Model file for the job. Use its own axes, mm. A direction names the side the tool comes from. Round coordinates to 2 decimals unless told otherwise and drop trailing zeros. Order: outer loops, then holes, each group sorted by start corner. A loop starts at its lowest first (then second) coordinate and runs counter-clockwise, first axis right, second up. Notation, with made-up numbers: (22, -23.75) -> (41, -23.75) arc R18 cw to (41, -7.75) -> close; hole circle Ø1 at (64.5, 57). An arc over 180 degrees is marked (long way). Put each result on its own line as item: value. Start each with the question number.
Q1. Pull direction Y, two halves, no side cores. Call faces 5 (the face through (-0.986, -4.714, -213.506)), 6 (the face through (44.15, 50.3, 3.4)), 7 (the face through (44.067, 47.942, 3.395)), 8 (the face through (-0.986, -4.714, 226.494)): released by +Y, released by -Y, zero draft, split by the parting line, or undercut.
Q2. Flat gauge pins, fed straight in: P1, Ø11, axis at x = 141.5, y = 69, coming from the +Z side; P2, Ø1.6, axis at y = 73.5, z = -232.5, coming from the +X side; P3, Ø15, axis at y = -5, z = 220, coming from the +X side. Where does each tip first touch, or does it go through?
Q3. Probe L1, parallel to Z at x = -0.85, y = -7.5; L2, parallel to X at y = 16.5, z = 79; L3, parallel to Y at x = -0.9, z = -220. List the from-to ranges inside material, lowest first.
Q4. Cut at B-B, the plane x = 121.5. List the corners of the cut face in (y, z).
Q5. Cut at A-A, the plane z = 148. List the corners of the cut face in (x, y).
Q6. Cut at C-C, the plane y = 38. List the corners of the cut face in (x, z).
Q7. 3-axis set-ups, long thin cutter, end or side, ignore diameter. For faces 1 (the face through (142.5, 67.9, -222.5)), 2 (the face through (0, -4, 3)), 3 (the face through (110, 72.152, 3)), 4 (the face through (142.5, 67.9, 222.5)): which of +Z, -Z, +X, -X, +Y, -Y reach the whole face in a straight line?
from build123d import *

# Parameters (mm, degrees)
BASIS_BLECH1_DEPTH               = 242.5
SKIZZE4_W                        = 22
SKIZZE4_H                        = 20
SCHNITT_LINEAR_AUSTRAGEN1_DEPTH  = 303.852114579
F_7_0_7_DURCHMESSER_BOHRUNG1_D   = 7
F_13_0_13_DURCHMESSER_BOHRUNG1_D = 13
F_7_0_7_DURCHMESSER_BOHRUNG2_D   = 7


# Sheet-metal steps are written as plain solids
with BuildPart() as part:
    # Skizze1 → Basis-Blech1 (new, symmetric)
    with BuildSketch(Plane.XY):
        with BuildLine():
            Line((0, -22.5), (0, 15.57179677))
            ThreePointArc((0, 15.57179677), (1.607695155, 21.57179677), (6, 25.964101615))
            Line((6, 25.964101615), (83.215390309, 70.544427996))
            ThreePointArc((83.215390309, 70.544427996), (86.109561768, 71.743233066), (89.215390309, 72.15212315))
            Line((89.215390309, 72.15212315), (132.216414533, 72.15212315))
            ThreePointArc((132.216414533, 72.15212315), (135.824884128, 71.596726559), (139.09933177, 69.981947682))
            Line((139.09933177, 69.981947682), (152.383040886, 60.680594423))
            Line((152.383040886, 60.680594423), (153.530193758, 62.318898512))
            Line((153.530193758, 62.318898512), (140.246484642, 71.62025177))
            ThreePointArc((140.246484642, 71.62025177), (136.426295727, 73.504160461), (132.216414533, 74.15212315))
            Line((132.216414533, 74.15212315), (89.215390309, 74.15212315))
            ThreePointArc((89.215390309, 74.15212315), (85.591923678, 73.675084718), (82.215390309, 72.276478803))
            Line((82.215390309, 72.276478803), (5, 27.696152423))
            ThreePointArc((5, 27.696152423), (-0.124355653, 22.57179677), (-2, 15.57179677))
            Line((-2, 15.57179677), (-2, -22.5))
            Line((-2, -22.5), (0, -22.5))
        make_face()
    extrude(amount=BASIS_BLECH1_DEPTH, both=True)

    # Skizze4 → Schnitt-Linear austragen1 (cut, through all)
    with BuildSketch(Plane(origin=(0, 74.15212315, 0), x_dir=(1, 0, 0), z_dir=(0, 1, 0))):
        with Locations((142.530193758, 232.5)):
            Rectangle(SKIZZE4_W, SKIZZE4_H)
        with Locations((142.530193758, -232.5)):
            Rectangle(SKIZZE4_W, SKIZZE4_H)
    extrude(amount=-SCHNITT_LINEAR_AUSTRAGEN1_DEPTH, mode=Mode.SUBTRACT)

    # Ø7.0 (7) Durchmesser Bohrung1 (through all)
    with Locations(Plane(origin=(-2, 72.15212315, 0), x_dir=(0, -1, 0), z_dir=(-1, 0, 0))):
        with Locations((79.65212315, 235), (79.65212315, -235)):
            Hole(F_7_0_7_DURCHMESSER_BOHRUNG1_D / 2)

    # Ø13.0 (13) Durchmesser Bohrung1 (through all)
    with Locations(Plane.ZY.offset(2)):
        with Locations((-220, -5), (220, -5)):
            Hole(F_13_0_13_DURCHMESSER_BOHRUNG1_D / 2)

    # Ø7.0 (7) Durchmesser Bohrung2 (through all)
    with Locations(Plane(origin=(79.790191976, 113.952203628, 0), x_dir=(0, 0, -1), z_dir=(0.5735764363510463, 0.8191520442889918, 0))):
        with Locations((0, -83.019920352), (-100, -83.019920352), (-200, -83.019920352), (100, -83.019920352), (200, -83.019920352)):
            Hole(F_7_0_7_DURCHMESSER_BOHRUNG2_D / 2)


solid = part.part
Ans:
1. face 5: undercut
1. face 6: released by +Y
1. face 7: released by -Y
1. face 8: undercut
2. P1: stops at z = 222.5
2. P2: stops at x = 131.53
2. P3: stops at x = 0
3. L1: z = -242.5 to -238.5, -231.5 to -226, -214 to 214, 226 to 231.5, 238.5 to 242.5
3. L2: x = -1.97 to 0.04
3. L3: y = -22.5 to -11.5, 1.5 to 21.01
4. outline: (72.15, -242.5) -> (74.15, -242.5) -> (74.15, 242.5) -> (72.15, 242.5) -> close
5. outline: (-2, -22.5) -> (0, -22.5) -> (0, 15.57) arc R12 cw to (6, 25.96) -> (83.22, 70.54) arc R12 cw to (89.22, 72.15) -> (132.22, 72.15) arc R12 cw to (139.1, 69.98) -> (152.38, 60.68) -> (153.53, 62.32) -> (140.25, 71.62) arc R14 ccw to (132.22, 74.15) -> (89.22, 74.15) arc R14 ccw to (82.22, 72.28) -> (5, 27.7) arc R14 ccw to (-2, 15.57) -> close
6. outline: (22.85, -242.5) -> (26.85, -242.5) -> (26.85, 242.5) -> (22.85, 242.5) -> close
7. face 1: -Z, +X, +Y, -Y
7. face 2: +Z, -Z, +X, -Y
7. face 3: +Z, -Z, -Y
7. face 4: +Z, +X, +Y, -Y
